Autodesk Inventor part; units mm, degrees
ref_plane "YZ Plane" through (0, 0, 0) normal (1, 0, 0) x (0, 1, 0)
ref_plane "XZ Plane" through (0, 0, 0) normal (0, 1, 0) x (-1, 0, 0)
ref_plane "XY Plane" through (0, 0, 0) normal (0, 0, 1) x (1, 0, 0)
sketch "Sketch1" plane through (0, 0, 0) normal (0, 1, 0) x (-1, 0, 0)
  circle A0 centre (0, 0) radius 609.6
  circle A1 centre (0, 0) radius 12.7
  circle A2 centre (0, 596.9) radius 2.6035
  line L0 (0, 12.7) -> (0, 594.2965)
  circle A3 centre (-596.9, 0) radius 2.6035
  circle A4 centre (0, -596.9) radius 2.6035
  circle A5 centre (596.9, 0) radius 2.6035
  point P0 (-594.2965, 0)
  point P1 (0, -594.2965)
  point P2 (594.2965, 0)
  dimension "d5" = 25.4
  dimension "d6" = 5.207
  dimension "d0" = 1219.2
  dimension "d7" = 596.9
  dimension "d10" = 360
extrude "Extrusion1" add sketch "Sketch1" along normal blind 19.05
properties part number "bottom" material "Wood (Birch)"
CAD build for the part. Positions are in the model's coordinates, mm. Give positions to 0.01 mm unless a question says otherwise; leave off trailing zeros. Write each loop counter-clockwise with the first axis right and the second up, starting at its lowest first coordinate (ties: lowest second). Pieces come first, ordered by that corner, then holes. Notation, with made-up numbers: M 6,43 L 52,43 A30 ccw 52,77 Z; hole C 68,-20.5 d11. An arc over 180 degrees is marked long. Return JSON: item names as keys, results as strings. Group by question number.
(1) Band-saw the part on C-C (z = 171). Give the cut face in (x, y).
(2) Drill centre lines: L1, parallel to Z at x = 0, y = 11.5; L2, parallel to Z at x = 15, y = 18.25; L3, parallel to X at y = 12.25, z = -13.5. Where is each one in solid material? Low to high. Write a range as [from, to].
(3) Band-saw the part on B-B (x = 357). Give the cut face in (y, z).
(4) Flat gauge pins, fed straight in: pin 1 Ø6 at (x, y) = (231, 5.5) entering from +Z; pin 2 Ø4 at (x, z) = (0, 596.9) entering from +Y; pin 3 Ø8 at (y, z) = (4, 426) entering from -X; pin 4 Ø8 at (x, y) = (166.5, 2) entering from +Z. Where does each tip first touch, or does it go through?
(5) Band-saw the part on A-A (y = 13.5). Give the cut face in (x, z).
Entries:
{
 "1": {"outline": "M -585.12,0 L 585.12,0 L 585.12,19.05 L -585.12,19.05 Z"},
 "2": {"L1": "z = [-609.6, -599.5], [-594.3, -12.7], [12.7, 594.3], [599.5, 609.6]", "L2": "z = [-609.42, 609.42]", "L3": "x = [-609.45, 609.45]"},
 "3": {"outline": "M 0,-494.13 L 19.05,-494.13 L 19.05,494.13 L 0,494.13 Z"},
 "4": {"pin 1": "stops at z = 565.36", "pin 2": "passes through", "pin 3": "stops at x = -439.92", "pin 4": "stops at z = 587.54"},
 "5": {"outline": "C 0,0 d1219.2; hole C -596.9,0 d5.21; hole C 0,0 d25.4; hole C 0,-596.9 d5.21; hole C 0,596.9 d5.21; hole C 596.9,0 d5.21"}
}
